Can you work these out from the drawing? Everything is in mm from the part's minimum corner. Round coordinates to 2 decimals unless told otherwise and drop trailing zeros. Order: outer loops, then holes, each group sorted by start corner. A loop starts at its lowest first (then second) coordinate and runs counter-clockwise, first axis right, second up. Notation, with made-up numbers: M -34.75,9.5 L 0.25,9.5 A23 ccw 0.25,38.5 Z; hole C 44.5,41.25 d7. An arc over 180 degrees is marked long. Write item = value, one per line. Start each with the question number.
Item 1: I'm going to push a flat-ended pin straight in: P1, Ø1.5, axis at x = 32, y = 8.5, coming from the +Z side. Where does the tip first touch, or does it pass through?
Item 2: Please list where these lines run through material, in increasing order: L1, parallel to Y at x = 19, z = 4.45; L2, parallel to Y at x = 2.5, z = 4.05.
Item 3: We'd pull the mould along Y, two halves only. Please class the marked faces 1, 2 and 3: pulls with the +Y half, pulls with the -Y half, needs draft (parallel to the pull), parting line crosses it, or undercut.
Item 4: I want a section at D-D, the plane y = 32.5. List the corners of the cut face in (x, z) for me, plus the area to 3 significant figures.
Item 5: I want a section at C-C, the plane y = 21. List the corners of the cut face in (x, z) for me.
Item 6: I want a section at B-B, the plane x = 36. List the corners of the cut face in (y, z) for me (3 decimals), plus the area to 3 significant figures.
Item 7: I want a section at A-A, the plane z = 4.15. State how many separate pieces and enclosed holes the cut face has, plus the area to 3 significant figures.
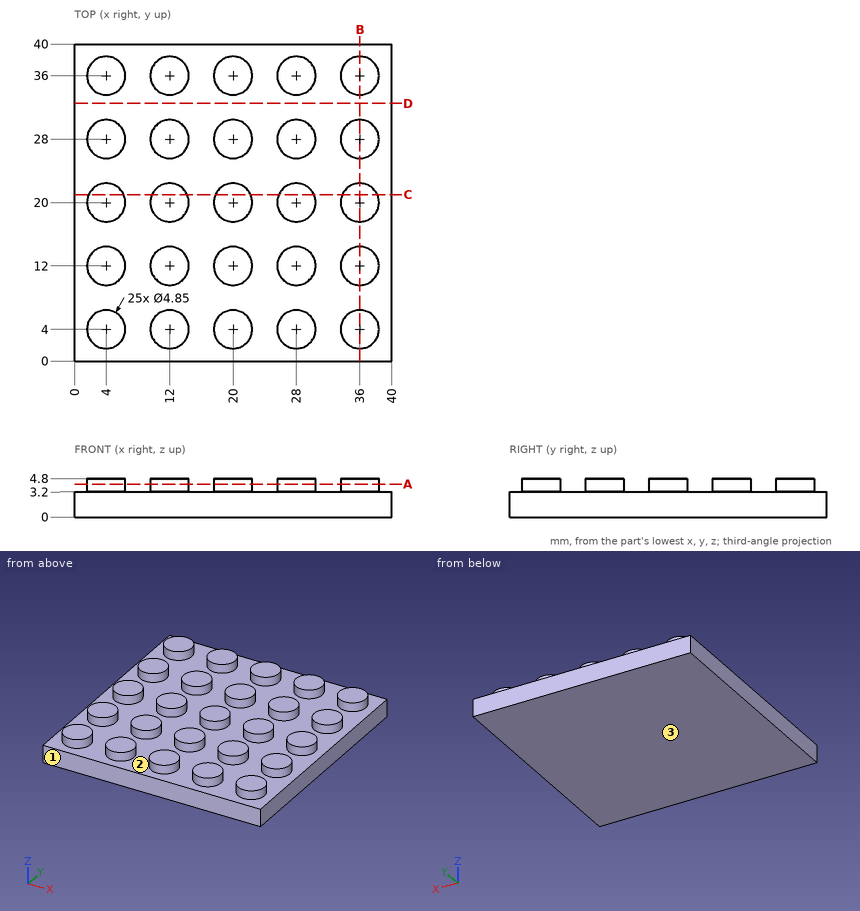
Filled in:
q1.P1 = 3.2
q2.L1 = 1.79 to 6.21, 9.79 to 14.21, 17.79 to 22.21, 25.79 to 30.21, 33.79 to 38.21
q2.L2 = 2.09 to 5.91, 10.09 to 13.91, 18.09 to 21.91, 26.09 to 29.91, 34.09 to 37.91
q3.face_1 = pulls with the -Y half
q3.face_2 = undercut
q3.face_3 = needs draft
q4.outline = M 0,0 L 40,0 L 40,3.2 L 0,3.2 Z
q4.area = 128 mm^2
q5.outline = M 0,0 L 40,0 L 40,3.2 L 38.21,3.2 L 38.21,4.8 L 33.79,4.8 L 33.79,3.2 L 30.21,3.2 L 30.21,4.8 L 25.79,4.8 L 25.79,3.2 L 22.21,3.2 L 22.21,4.8 L 17.79,4.8 L 17.79,3.2 L 14.21,3.2 L 14.21,4.8 L 9.79,4.8 L 9.79,3.2 L 6.21,3.2 L 6.21,4.8 L 1.79,4.8 L 1.79,3.2 L 0,3.2 Z
q6.outline = M 0,0 L 40,0 L 40,3.2 L 38.425,3.2 L 38.425,4.8 L 33.575,4.8 L 33.575,3.2 L 30.425,3.2 L 30.425,4.8 L 25.575,4.8 L 25.575,3.2 L 22.425,3.2 L 22.425,4.8 L 17.575,4.8 L 17.575,3.2 L 14.425,3.2 L 14.425,4.8 L 9.575,4.8 L 9.575,3.2 L 6.425,3.2 L 6.425,4.8 L 1.575,4.8 L 1.575,3.2 L 0,3.2 Z
q6.area = 167 mm^2
q7.separate_pieces = 25
q7.enclosed_holes = 0
q7.area = 462 mm^2
